The listing builds one solid part. Answer for the finished solid, in the listing's coordinates (mm). Face numbers are marked on the shaded views. A direction names the side the tool comes from. Round coordinates to 2 decimals unless told otherwise and drop trailing zeros. Loops run counter-clockwise (first coordinate to the right, second up) from the corner with the lowest first, then second, coordinate; pieces in that order, holes last. Notation, with made-up numbers: M 13.25,7.25 L 44.25,7.25 A23 cw 44.25,25.25 Z; hole C 60,-30 d6. An arc over 180 degrees is marked long. Answer as a JSON object with one key per item and string values.
```python
from build123d import *

# Parameters (mm, degrees)
BOSS_EXTRUDE1_DEPTH = 50
BOSS_EXTRUDE2_DEPTH = 10
SKETCH4_R           = 5
CUT_EXTRUDE1_DEPTH  = 10
SKETCH5_R           = 5
CUT_EXTRUDE2_DEPTH  = 10
SKETCH6_R           = 5
CUT_EXTRUDE3_DEPTH  = 10


with BuildPart() as part:
    # Sketch1 → Boss-Extrude1 (new body)
    with BuildSketch(Plane.XY):
        Polygon((0, 110), (10, 110), (10, 10), (60, 10), (60, 0), (0, 0), align=None)
    extrude(amount=BOSS_EXTRUDE1_DEPTH)

    # Sketch2 → Boss-Extrude2 (add)
    with BuildSketch(Plane.XY.offset(50)):
        Polygon((0, 110), (35, 110), (35, 35), (60, 35), (60, 0), (0, 0), align=None)
    extrude(amount=BOSS_EXTRUDE2_DEPTH)

    # Sketch4 → Cut-Extrude1 (cut)
    with BuildSketch(Plane(origin=(10, 0, 0), x_dir=(0, 0, -1), z_dir=(1, 0, 0))):
        with Locations((-25, 60)):
            Circle(SKETCH4_R)
        with Locations((-25, 85)):
            Circle(SKETCH4_R)
        with Locations((-25, 35)):
            Circle(SKETCH4_R)
    extrude(amount=-CUT_EXTRUDE1_DEPTH, mode=Mode.SUBTRACT)

    # Sketch5 → Cut-Extrude2 (cut)
    with BuildSketch(Plane(origin=(0, 10, 0), x_dir=(1, 0, 0), z_dir=(0, 1, 0))):
        with Locations(Location((45, -25, 0), (0, 0, 270))):
            Circle(SKETCH5_R)
        with Locations(Location((25, -25, 0), (0, 0, 270))):
            Circle(SKETCH5_R)
    extrude(amount=-CUT_EXTRUDE2_DEPTH, mode=Mode.SUBTRACT)

    # Sketch6 → Cut-Extrude3 (cut)
    with BuildSketch(Plane(origin=(0, 0, 50), x_dir=(-1, 0, 0), z_dir=(0, 0, -1))):
        with Locations((-22.5, 22.5)):
            Circle(SKETCH6_R)
        with Locations((-22.5, 55)):
            Circle(SKETCH6_R)
        with Locations((-22.5, 90)):
            Circle(SKETCH6_R)
        with Locations((-45, 22.5)):
            Circle(SKETCH6_R)
    extrude(amount=-CUT_EXTRUDE3_DEPTH, mode=Mode.SUBTRACT)


solid = part.part
```
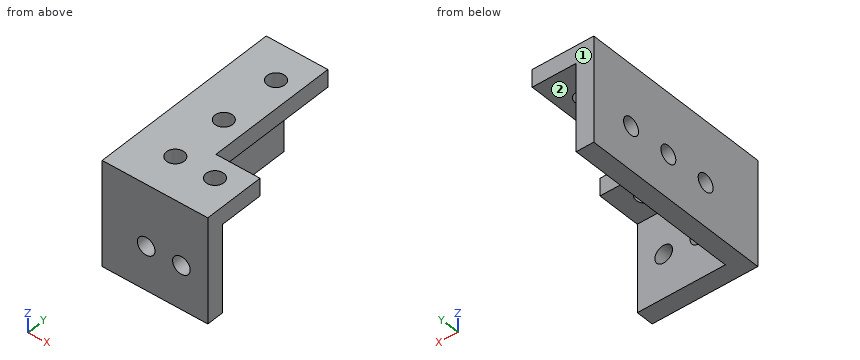
Item 1: Flat-ended cylindrical pins translate along their axes: P1, Ø5, axis at x = 48.5, z = 53, coming from the +Y side; P2, Ø9, axis at x = 22.5, y = 90, coming from the -Z side; P3, Ø13, axis at x = 45, y = 22.5, coming from the -Z side; P4, Ø12, axis at y = 96, z = 14, coming from the +X side. Find the tip coordinate at first contact, or state that the pin passes through.
Values follow:
{"P1": "y = 35", "P2": "through", "P3": "z = 50", "P4": "x = 10"}
Item 2: Straight lines are drawn through the part: line 1 (X direction, y = 3, z = 25); line 2 (Y direction, x = 22, z = 53); line 3 (Y direction, x = 45, z = 55.5). For each, find the intervals that lie inside material, in ascending order.
Values follow:
{"line 1": "0 to 20, 30 to 40, 50 to 60", "line 2": "0 to 17.53, 27.47 to 50.03, 59.97 to 85.03, 94.97 to 110", "line 3": "0 to 17.5, 27.5 to 35"}
Item 3: The part is cut by section C-C (x = 25). Give the vertices of the cut face in (y, z).
Values follow:
{"outline": "M 0,0 L 10,0 L 10,20 L 0,20 Z; M 0,30 L 10,30 L 10,50 L 18.17,50 L 18.17,60 L 0,60 Z; M 26.83,50 L 50.67,50 L 50.67,60 L 26.83,60 Z; M 59.33,50 L 85.67,50 L 85.67,60 L 59.33,60 Z; M 94.33,50 L 110,50 L 110,60 L 94.33,60 Z"}
Item 4: Which of the six approach directions +Z, -Z, +X, -X, +Y, -Y give full straight-line access (tool end or side, diameter ignored) to the marked faces 1 and 2?
Values follow:
{"face 1": "+Z, -Z, +X, -X, +Y", "face 2": "-Z, +X, +Y"}
Item 5: The part is cut by section A-A (y = 22.5). Give the vertices of the cut face in (x, z).
Values follow:
{"outline": "M 0,0 L 10,0 L 10,50 L 17.5,50 L 17.5,60 L 0,60 Z; M 27.5,50 L 40,50 L 40,60 L 27.5,60 Z; M 50,50 L 60,50 L 60,60 L 50,60 Z"}
Item 6: The part is cut by section D-D (z = 18). Give the vertices of the cut face in (x, y).
Values follow:
{"outline": "M 0,0 L 60,0 L 60,10 L 10,10 L 10,110 L 0,110 Z"}
Item 7: The part is cut by section B-B (x = 46.5). Give the vertices of the cut face in (y, z).
Values follow:
{"outline": "M 0,0 L 10,0 L 10,20.23 L 0,20.23 Z; M 0,29.77 L 10,29.77 L 10,50 L 17.73,50 L 17.73,60 L 0,60 Z; M 27.27,50 L 35,50 L 35,60 L 27.27,60 Z"}
